Here's how the part is built. I have some questions about the finished solid (model axes, mm). Coordinates: 2 decimals unless noted, no trailing zeros. Write each loop counter-clockwise with the first axis right and the second up, starting at its lowest first coordinate (ties: lowest second). Pieces come first, ordered by that corner, then holes. Notation, with made-up numbers: (18, 35.25) -> (45, 35.25) arc R19 cw to (45, 47.25) -> close; hole circle Ø9 at (37, -2). An arc over 180 degrees is marked (long way). Use a Markdown table: item, result. Add a question column.
Item 1: If I drill on line 1 along X through (y, z) = (1.25, 73); line 2 along Y through (x, z) = (15.5, 62); line 3 along Y through (x, z) = (4.25, 91.5), over which ranges is the centre line in solid material (lowest first)? Write a range as from..to.
Item 2: Will these pins go through, and if not, where does the flat tip stop? pin 1 Ø2 at (x, z) = (10.5, 75) entering from +Y; pin 2 Ø2 at (y, z) = (10.5, 60.5) entering from +X; pin 3 Ø4.5 at (y, z) = (9.5, 45) entering from -X; pin 4 Ø2.5 at (x, y) = (10, 10) entering from +Z (3 decimals).
Item 3: Imagine slicing it at A-A, the plane x = 10. Write out the boundary of the cut face in (y, z), and give its area (3 significant figures).
Item 4: Imagine slicing it at C-C, the plane x = 15. Write out the boundary of the cut face in (y, z).
```python
from build123d import *

# Parameters (mm, degrees)
SKETCH1_W           = 8
SKETCH1_H           = 8
SKETCH1_R           = 2.1
BOSS_EXTRUDE1_DEPTH = 100


with BuildPart() as part:
    # Sketch1 → Boss-Extrude1 (new body)
    # profile 1 of 5: a face of its own
    with BuildSketch(Plane.XY):
        Polygon((2, 16), (6, 12), (6, 14), (8, 14), (4, 18), (7, 18), (7, 20), (0, 20), (0, 13), (2, 13), align=None)
    # profile 2 of 5: a face of its own
    with BuildSketch(Plane.XY):
        Polygon((16, 18), (12, 14), (14, 14), (14, 12), (18, 16), (18, 13), (20, 13), (20, 20), (13, 20), (13, 18), align=None)
    # profile 3 of 5: a face of its own
    with BuildSketch(Plane.XY):
        with Locations((10, 10)):
            Rectangle(SKETCH1_W, SKETCH1_H)
        with Locations((10, 10)):
            Circle(SKETCH1_R, mode=Mode.SUBTRACT)
    # profile 4 of 5: a face of its own
    with BuildSketch(Plane.XY):
        Polygon((6, 8), (2, 4), (2, 7), (0, 7), (0, 0), (7, 0), (7, 2), (4, 2), (8, 6), (6, 6), align=None)
    # profile 5 of 5: a face of its own
    with BuildSketch(Plane.XY):
        Polygon((14, 6), (12, 6), (16, 2), (13, 2), (13, 0), (20, 0), (20, 7), (18, 7), (18, 4), (14, 8), align=None)
    extrude(amount=BOSS_EXTRUDE1_DEPTH)


solid = part.part
```
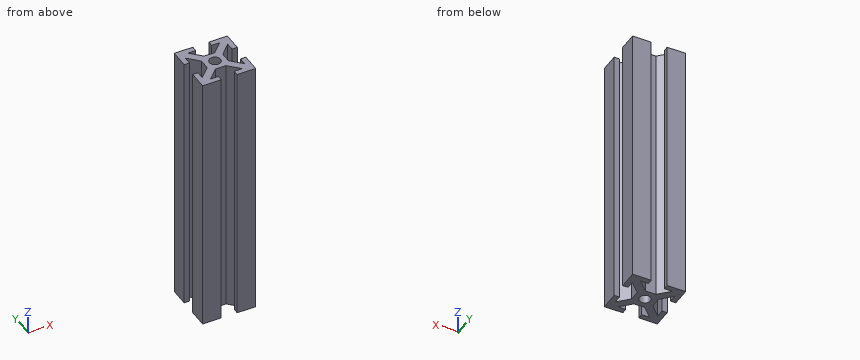
Ans:
| question | item | result |
|---|---|---|
| 1 | line 1 | x = 0..7, 13..20 |
| 1 | line 2 | y = 0..2, 2.5..6.5, 13.5..17.5, 18..20 |
| 1 | line 3 | y = 0..2, 2.25..6.25, 13.75..17.75, 18..20 |
| 2 | pin 1 | stops at y = 14 |
| 2 | pin 2 | stops at x = 14 |
| 2 | pin 3 | stops at x = 5.25 |
| 2 | pin 4 | passes through |
| 3 | outline | (6, 0) -> (7.9, 0) -> (7.9, 100) -> (6, 100) -> close; (12.1, 0) -> (14, 0) -> (14, 100) -> (12.1, 100) -> close |
| 3 | area | 380 mm^2 |
| 4 | outline | (0, 0) -> (2, 0) -> (2, 100) -> (0, 100) -> close; (3, 0) -> (7, 0) -> (7, 100) -> (3, 100) -> close; (13, 0) -> (17, 0) -> (17, 100) -> (13, 100) -> close; (18, 0) -> (20, 0) -> (20, 100) -> (18, 100) -> close |
